Can you work these out from the model? Positions are in its coordinate system, mm. A direction names the side the tool comes from. Coordinates: 2 decimals unless noted, no trailing zeros. Order: outer loops, then holes, each group sorted by start corner. A loop starts at its lowest first (then second) coordinate and runs counter-clockwise, first axis right, second up. Notation, with made-up numbers: (83, 19.5) -> (111, 19.5) arc R35 cw to (111, 54.5) -> close; hole circle Ø5 at (23.5, -14.75). An arc over 180 degrees is marked (long way). Answer in a Markdown table with one row per item. Add a question column.
1. Imagine slicing it at C-C on y = 14. Write out the boundary of the cut face in (x, z), plus the area to 3 significant figures.
2. Imagine slicing it at B-B on z = 2.5. State how many separate pieces and enclosed holes the cut face has, plus the area to 3 significant figures.
3. Will these pins go through, and if not, where does the flat tip stop? pin 1 (4 mm diameter, centred on x = -29.37, z = 19, fed in from +Y); pin 2 (4.5 mm diameter, centred on y = -20.5, z = 11.5, fed in from -X); pin 3 (11 mm diameter, centred on x = -9, y = -7, fed in from +Z).
4. We'd pull the mould along X, two halves only. Please class faces 1 (the face through (30.6, -19.5, 20.1)), 2 (the face through (1, -17.5, 14)), 3 (the face through (-56, 8, 2)): pulls with the +X half, pulls with the -X half, needs draft (parallel to the pull), parting line crosses it, or undercut.
5. Imagine slicing it at D-D on x = 16.5. Write out the boundary of the cut face in (y, z).
6. Imagine slicing it at A-A on y = 7.5. Write out the boundary of the cut face in (x, z), plus the area to 3 significant figures.
7. If I drill on line 1 along Z through (x, y) = (25, -12.5); line 2 along X through (y, z) = (-18, 13); line 3 along Y through (x, z) = (-14, 16.75), over which ranges is the centre line in solid material (lowest first)? Write a range as [from, to].
8. On a 3-axis mill with a long thin cutter (end or side, diameter ignored), from which of +Z, -Z, +X, -X, +Y, -Y can I reach the whole of each face in a straight line? I mean faces 4 (the face through (-28.058, -19.472, 4.996)), 5 (the face through (35.368, -20, 16)), 6 (the face through (-1, -4, 4)), 7 (the face through (0, -19, 25)), 8 (the face through (39.704, 17, 2)). Say none if no direction works.
from build123d import *

# Parameters (mm, degrees)
F0_R     = 2.5
F0_R_2   = 2
F1_DEPTH = 4
F3_DEPTH = 21
F5_DEPTH = 25
F6_D     = 3.3
F7_SIZE  = 2


# Not quite as in the source:
# - ends of sketch curves that miss each other by under 0.0002 mm in the source are joined


with BuildPart() as f1:
    # F0 (on Top) → F1 (new body)
    with BuildSketch(Plane.XY):
        with BuildLine():
            ThreePointArc((0, 18.5), (13.081475452, 13.081475452), (18.5, 0))
            ThreePointArc((18.5, 0), (-1.1345020789, -18.4651808828), (-18.3608545982, 2.2647336323))
            ThreePointArc((-18.3608545982, 2.2647336323), (-20.315445832, 5.8895882396), (-20.061448931, 9.9999998237))
            ThreePointArc((-20.061448931, 9.9999998237), (-38.4593739655, 0.6163893281), (-48.7895366382, 18.5))
            Line((-48.7895366382, 18.5), (-55, 18.5))
            Line((-55, 18.5), (-55, -3.5))
            Line((-55, -3.5), (-35, -20.5))
            Line((-35, -20.5), (0, -20.5))
            Line((0, -20.5), (35, -20.5))
            Line((35, -20.5), (55, -3.5))
            Line((55, -3.5), (55, 18.5))
            Line((55, 18.5), (39.703517094, 18.5))
            Line((39.703517094, 18.5), (39.703517094, 15))
            ThreePointArc((39.703517094, 15), (39.7035676427, 14.9863858353), (39.703517094, 14.9727717541))
            ThreePointArc((39.703517094, 14.9727717541), (34.1416723213, 9.5003484762), (28.7044327696, 15.096593634))
            Line((28.7044327696, 15.096593634), (28.7642142424, 18.5))
            Line((28.7642142424, 18.5), (0, 18.5))
        make_face()
        with BuildLine():
            ThreePointArc((-18.3608545982, 2.2647336323), (-1.1345020789, -18.4651808828), (18.5, 0))
            ThreePointArc((18.5, 0), (13.081475452, 13.081475452), (0, 18.5))
            ThreePointArc((0, 18.5), (-5.8749853417, 17.542364357), (-11.1417441574, 14.7685997011))
            ThreePointArc((-11.1417441574, 14.7685997011), (-7.0694530575, 12.1035433774), (-5.4903810568, 7.5))
            ThreePointArc((-5.4903810568, 7.5), (-5.7459373553, 5.5588571779), (-6.4951905116, 3.750000029))
            ThreePointArc((-6.4951905116, 3.750000029), (-12.0588494406, 0.0580749232), (-18.3608545982, 2.2647336323))
        make_face()
        with BuildLine():
            ThreePointArc((7.5, 0), (-1.9411428544, -7.2444436928), (-6.4951905116, 3.750000029))
            ThreePointArc((-6.4951905116, 3.750000029), (1.9411428544, 7.2444436928), (7.5, 0))
        make_face(mode=Mode.SUBTRACT)
        with BuildLine():
            ThreePointArc((7.5, 0), (1.9411428544, 7.2444436928), (-6.4951905116, 3.750000029))
            ThreePointArc((-6.4951905116, 3.750000029), (-1.9411428544, -7.2444436928), (7.5, 0))
        make_face()
        Circle(F0_R, mode=Mode.SUBTRACT)
        with BuildLine():
            ThreePointArc((-11.1417441574, 14.7685997011), (-16.02146997, 9.25), (-18.3608545982, 2.2647336323))
            ThreePointArc((-18.3608545982, 2.2647336323), (-12.0588494406, 0.0580749232), (-6.4951905116, 3.750000029))
            ThreePointArc((-6.4951905116, 3.750000029), (-5.7459373553, 5.5588571779), (-5.4903810568, 7.5))
            ThreePointArc((-5.4903810568, 7.5), (-7.0694530575, 12.1035433774), (-11.1417441574, 14.7685997011))
        make_face()
        with Locations((-12.9903810568, 7.5)):
            Circle(F0_R_2, mode=Mode.SUBTRACT)
        with BuildLine():
            ThreePointArc((-20.061448931, 9.9999998237), (-20.315445832, 5.8895882396), (-18.3608545982, 2.2647336323))
            ThreePointArc((-18.3608545982, 2.2647336323), (-16.02146997, 9.25), (-11.1417441574, 14.7685997011))
            ThreePointArc((-11.1417441574, 14.7685997011), (-16.5263862207, 14.1141263581), (-20.061448931, 9.9999998237))
        make_face()
        with BuildLine():
            ThreePointArc((-11.1417441574, 14.7685997011), (-5.8749853417, 17.542364357), (0, 18.5))
            Line((0, 18.5), (-19.6176323465, 18.5))
            ThreePointArc((-19.6176323465, 18.5), (-19.3074560996, 16.7622028562), (-19.2035844924, 15))
            ThreePointArc((-19.2035844924, 15), (-19.4196061134, 12.463470227), (-20.061448931, 9.9999998237))
            ThreePointArc((-20.061448931, 9.9999998237), (-16.5263862207, 14.1141263581), (-11.1417441574, 14.7685997011))
        make_face()
        with BuildLine():
            ThreePointArc((-19.2035844924, 15), (-19.3074560996, 16.7622028562), (-19.6176323465, 18.5))
            Line((-19.6176323465, 18.5), (-28.7642142424, 18.5))
            Line((-28.7642142424, 18.5), (-28.7044327696, 15.096593634))
            ThreePointArc((-28.7044327696, 15.096593634), (-28.7037965658, 15.0482986794), (-28.7035844924, 15))
            ThreePointArc((-28.7035844924, 15), (-34.1899703277, 9.5000168496), (-39.703517094, 14.9727717541))
            Line((-39.703517094, 14.9727717541), (-39.703517094, 18.5))
            Line((-39.703517094, 18.5), (-48.7895366382, 18.5))
            ThreePointArc((-48.7895366382, 18.5), (-38.4593739655, 0.6163893281), (-20.061448931, 9.9999998237))
            ThreePointArc((-20.061448931, 9.9999998237), (-19.4196061134, 12.463470227), (-19.2035844924, 15))
        make_face()
        Polygon((-55, -3.5), (-55, 18.5), (-56, 18.5), (-56, -3.9624404748), (-35.3675770292, -21.5), (0, -21.5), (35.3675770292, -21.5), (56, -3.9624404748), (56, 18.5), (55, 18.5), (55, -3.5), (35, -20.5), (0, -20.5), (-35, -20.5), align=None)
    extrude(amount=F1_DEPTH)

    # F2 (on face) → F3 (join)
    with BuildSketch(Plane.XY.offset(4)):
        Polygon((40.0734593822, -17.5), (-40.0734593822, -17.5), (-35.3675770292, -21.5), (35.3675770292, -21.5), align=None)
    extrude(amount=F3_DEPTH)

    # F4 (on face) → F5 (cut)
    with BuildSketch(Plane.XZ.offset(21.5)):
        with BuildLine():
            Line((-35.3675770292, 25), (-40.0734593822, 25))
            Line((-40.0734593822, 25), (-40.0734593822, 4))
            Line((-40.0734593822, 4), (-38.3675770292, 4))
            ThreePointArc((-38.3675770292, 4), (-36.2462566857, 4.8786796564), (-35.3675770292, 7))
            Line((-35.3675770292, 7), (-35.3675770292, 25))
        make_face()
        with BuildLine():
            Line((40.0734593822, 25), (35.3675770292, 25))
            Line((35.3675770292, 25), (35.3675770292, 7))
            ThreePointArc((35.3675770292, 7), (36.2462566857, 4.8786796564), (38.3675770292, 4))
            Line((38.3675770292, 4), (40.0734593822, 4))
            Line((40.0734593822, 4), (40.0734593822, 25))
        make_face()
    extrude(amount=-F5_DEPTH, mode=Mode.SUBTRACT)

    # F6 (through all)
    with Locations(Plane.XZ.offset(21.5)):
        with Locations((-29.3675770292, 19), (-29.3675770292, 6), (29.3675770292, 6), (29.3675770292, 19)):
            Hole(F6_D / 2)

    # F7
    f7_edges = [f1.edges().sort_by_distance(p)[0] for p in [
        (-56, -3.96244, 2),
        (56, -3.96244, 2),
    ]]
    chamfer(f7_edges, length=F7_SIZE)


solid = f1.part
Answers follow:
| question | item | result |
|---|---|---|
| 1 | outline | (-56, 0) -> (-39.61, 0) -> (-39.61, 4) -> (-56, 4) -> close; (-28.8, 0) -> (28.8, 0) -> (28.8, 4) -> (-28.8, 4) -> close; (39.61, 0) -> (56, 0) -> (56, 4) -> (39.61, 4) -> close |
| 1 | area | 361 mm² |
| 2 | separate pieces | 1 |
| 2 | enclosed holes | 2 |
| 2 | area | 3,910 mm² |
| 3 | pin 1 | stops at y = -17.5 |
| 3 | pin 2 | stops at x = -35.37 |
| 3 | pin 3 | stops at z = 4 |
| 4 | face 1 | undercut |
| 4 | face 2 | needs draft |
| 4 | face 3 | pulls with the -X half |
| 5 | outline | (-21.5, 0) -> (18.5, 0) -> (18.5, 4) -> (-17.5, 4) -> (-17.5, 25) -> (-21.5, 25) -> close |
| 6 | outline | (-56, 0) -> (-14.99, 0) -> (-14.99, 4) -> (-56, 4) -> close; (-10.99, 0) -> (56, 0) -> (56, 4) -> (-10.99, 4) -> close |
| 6 | area | 432 mm² |
| 7 | line 1 | z = [0, 4] |
| 7 | line 2 | x = [-35.37, 35.37] |
| 7 | line 3 | y = [-21.5, -17.5] |
| 8 | face 4 | +Y, -Y |
| 8 | face 5 | +Z, +X, +Y, -Y |
| 8 | face 6 | +Z, +X, -X, +Y |
| 8 | face 7 | +Z, +X, -X, +Y, -Y |
| 8 | face 8 | +Z, -Z, +Y |
